Input: dimensioned drawing with shaded views. Units: mm. Origin: part minimum x, y, z. Give positions to 0.01 mm unless a question says otherwise; leave off trailing zeros. Loops run counter-clockwise (first coordinate to the right, second up) from the corner with the lowest first, then second, coordinate; pieces in that order, holes last.
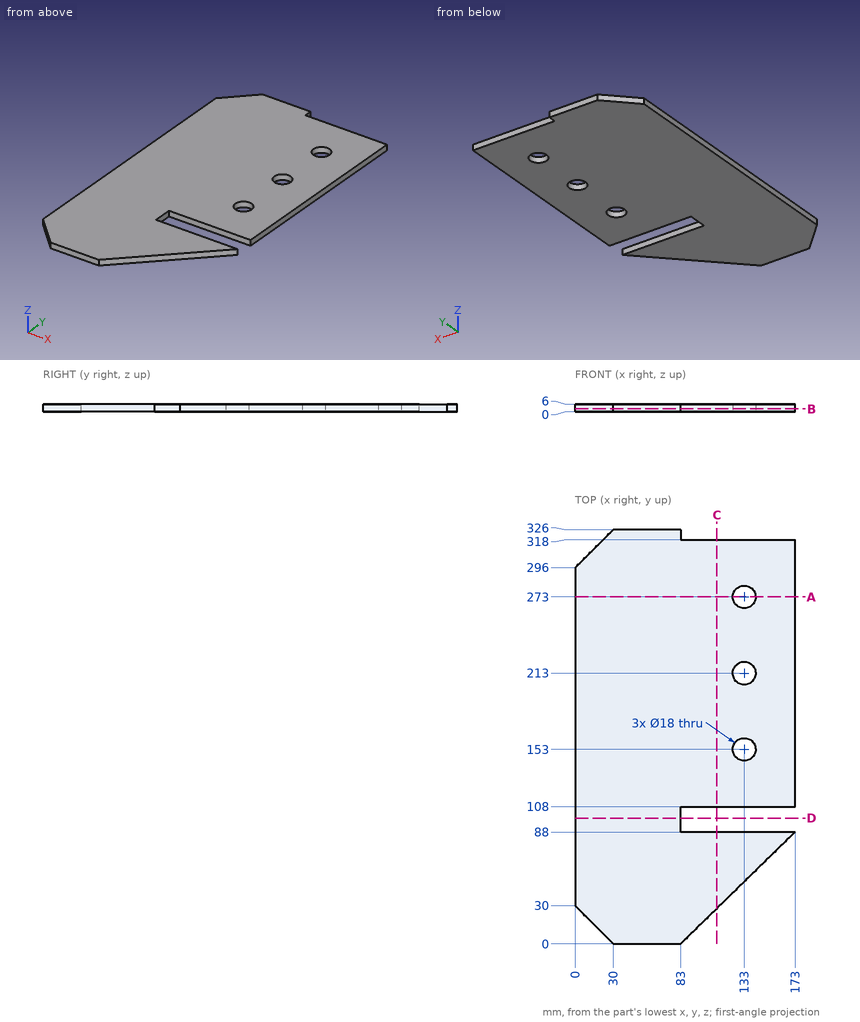
Item 1: Section query B-B on z = 2.2. Return loops of the section in (x, y), plus the area to 3 significant figures.
Values follow:
outline: (0, 30) - (30, 0) - (83, 0) - (173, 88) - (83, 88) - (83, 108) - (173, 108) - (173, 318) - (83, 318) - (83, 326) - (30, 326) - (0, 296) - close; hole circle Ø18 at (133, 153); hole circle Ø18 at (133, 213); hole circle Ø18 at (133, 273)
area: 48,300 mm2
Item 2: Section query C-C on x = 111.5. Return loops of the section in (y, z), plus the area to 3 significant figures.
Values follow:
outline: (27.87, 0) - (88, 0) - (88, 6) - (27.87, 6) - close; (108, 0) - (318, 0) - (318, 6) - (108, 6) - close
area: 1,620 mm2
Item 3: Section query D-D on y = 99. Return loops of the section in (x, z).
Values follow:
outline: (0, 0) - (83, 0) - (83, 6) - (0, 6) - close
Item 4: Ray query, probe 1 along X at (y, z) = (153, 1.75); probe 2 along Y at (x, z) = (137, 2.9); probe 3 along Y at (x, z) = (139, 2.7). Return the intervals inside material, ascending.
Values follow:
probe 1: x = 0 to 124, 142 to 173
probe 2: y = 52.8 to 88, 108 to 144.94, 161.06 to 204.94, 221.06 to 264.94, 281.06 to 318
probe 3: y = 54.76 to 88, 108 to 146.29, 159.71 to 206.29, 219.71 to 266.29, 279.71 to 318
Item 5: Pin query (flat end, axial travel): pin 1 (2 mm diameter, centred on x = 149.5, z = 1.5, fed in from +Y); pin 2 (1.8 mm diameter, centred on y = 320, z = 3.5, fed in from +X); pin 3 (10 mm diameter, centred on x = 122.5, y = 286, fed in from -Z). Return the tip coordinate at first contact, or that it passes through.
Values follow:
pin 1: stops at y = 318
pin 2: stops at x = 83
pin 3: stops at z = 0
Item 6: Section query A-A on y = 273. Return loops of the section in (x, z), plus the area to 3 significant figures.
Values follow:
outline: (0, 0) - (124, 0) - (124, 6) - (0, 6) - close; (142, 0) - (173, 0) - (173, 6) - (142, 6) - close
area: 930 mm2
